```python
from build123d import *

# Parameters (mm, degrees)
BOSS_EXTRUDE2_DEPTH = 3
SKETCH4_R           = 3
CUT_EXTRUDE2_DEPTH  = 2.5


with BuildPart() as part:
    # Sketch1 → Boss-Extrude2 (new body, symmetric)
    with BuildSketch(Plane(origin=(0, 0, 0), x_dir=(1, 0, 0), z_dir=(0, 1, 0))):
        with BuildLine():
            ThreePointArc((5, 0), (-3.535533906, 3.535533906), (0, -5))
            Line((0, -5), (20, -5))
            ThreePointArc((20, -5), (27.071067812, -2.071067812), (30, 5))
            ThreePointArc((30, 5), (27.5, 7.5), (25, 5))
            ThreePointArc((25, 5), (23.535533906, 1.464466094), (20, 0))
            Line((20, 0), (5, 0))
        make_face()
    extrude(amount=BOSS_EXTRUDE2_DEPTH, both=True)

    # Sketch4 → Cut-Extrude2 (cut)
    with BuildSketch(Plane.XZ.offset(3)):
        Circle(SKETCH4_R)
    extrude(amount=-CUT_EXTRUDE2_DEPTH, mode=Mode.SUBTRACT)


solid = part.part
```
Design review of the part built by this model. Coordinates are the model's own, in mm. A direction names the side the tool comes from. Give positions to 0.01 mm unless a question says otherwise; leave off trailing zeros. Loops run counter-clockwise (first coordinate to the right, second up) from the corner with the lowest first, then second, coordinate; pieces in that order, holes last. Notation, with made-up numbers: (23.25, -27.75) -> (35.25, -27.75) arc R15 ccw to (35.25, -11.75) -> close; hole circle Ø7 at (-19.75, 82.25). An arc over 180 degrees is marked (long way). One line per item, written item: value.
Q1. For pin 1 Ø5 at (x, z) = (0, 0) entering from -Y; pin 2 Ø2 at (x, y) = (23.5, -2.5) entering from +Z; pin 3 Ø1.5 at (y, z) = (-2.5, -1.5) entering from +X, all flat-tipped, find the tip position at first contact; note any pin that passes through.
Numbers:
pin 1: stops at y = -0.5
pin 2: stops at z = 4.68
pin 3: stops at x = 29.61
Q2. Machinability: for faces 1 (the cylindrical face through (-3, -2, 0)), 2 (the cylindrical face through (24, 0, -2)), 3 (the flat face through (10, 0, 5)), which of the approach directions +Z, -Z, +X, -X, +Y, -Y give a long, thin tool a straight path to every point of the face, cutting with its end or side? Answer none if there is none.
Numbers:
face 1: -Y
face 2: -Z, +Y, -Y
face 3: +Z, +X, -X, +Y, -Y
Q3. We need section C-C on y = 0.4. Give the boundary of the cut face in (x, z).
Numbers:
outline: (0, 5) arc R5 ccw (long way) to (5, 0) -> (20, 0) arc R5 cw to (25, -5) arc R2.5 ccw to (30, -5) arc R10 ccw to (20, 5) -> close
Q4. We need section A-A on y = -1.6. Give the boundary of the cut face in (x, z), and give its area (3 significant figures).
Numbers:
outline: (0, 5) arc R5 ccw (long way) to (5, 0) -> (20, 0) arc R5 cw to (25, -5) arc R2.5 ccw to (30, -5) arc R10 ccw to (20, 5) -> close; hole circle Ø6 at (0, 0)
area: 199 mm^2
Q5. Draft analysis for pull direction Z (two halves, no side actions). For faces 4 (the flat face through (0, -0.5, 0)), 5 (the cylindrical face through (27.6, 0, -7.5)), 6 (the flat face through (12, 3, 1)), state which applies: pulls with the +Z half, pulls with the -Z half, needs draft (parallel to the pull), parting line crosses it, or undercut.
Numbers:
face 4: undercut
face 5: pulls with the -Z half
face 6: needs draft
Q6. We need section B-B on z = -4.5. Give the boundary of the cut face in (x, y), and give its area (3 significant figures).
Numbers:
outline: (-2.18, -3) -> (2.18, -3) -> (2.18, 3) -> (-2.18, 3) -> close; (24.97, -3) -> (29.99, -3) -> (29.99, 3) -> (24.97, 3) -> close
area: 56.2 mm^2
Q7. We need section D-D on z = 1. Give the boundary of the cut face in (x, y).
Numbers:
outline: (-4.9, -3) -> (-2.83, -3) -> (-2.83, -0.5) -> (2.83, -0.5) -> (2.83, -3) -> (28, -3) -> (28, 3) -> (-4.9, 3) -> close
Q8. For L1, parallel to Z at x = 0, y = -1.6; L2, parallel to Z at x = 6.5, y = 0.9; L3, parallel to Y at x = -0.5, z = -2, list the stretches that pass through material, from the lowest coordinate up.
Numbers:
L1: z = -5 to -3, 3 to 5
L2: z = 0 to 5
L3: y = -0.5 to 3
